CAD build for the part. Positions are in the model's coordinates, mm. Round coordinates to 2 decimals unless told otherwise and drop trailing zeros. Order: outer loops, then holes, each group sorted by start corner. A loop starts at its lowest first (then second) coordinate and runs counter-clockwise, first axis right, second up. Notation, with made-up numbers: (17.5, -32.75) - (31.5, -32.75) arc R21 cw to (31.5, -5.75) - close; hole circle Ø8 at (23, 6). An arc over 180 degrees is marked (long way). Use one line per item in the form item = value. Start each with the question number.
from build123d import *

# Parameters (mm, degrees)
SKETCH3_W           = 152.4
SKETCH3_H           = 152.4
BOSS_EXTRUDE1_DEPTH = 3.175
SKETCH4_R           = 11
CUT_EXTRUDE1_DEPTH  = 10
SKETCH5_R           = 3.175
CUT_EXTRUDE5_DEPTH  = 10


with BuildPart() as part:
    # Sketch3 → Boss-Extrude1 (new, symmetric)
    with BuildSketch(Plane(origin=(0, 0, 0), x_dir=(1, 0, 0), z_dir=(0, 1, 0))):
        Rectangle(SKETCH3_W, SKETCH3_H)
    extrude(amount=BOSS_EXTRUDE1_DEPTH, both=True)

    # Sketch4 → Cut-Extrude1 (cut)
    with BuildSketch(Plane(origin=(0, 3.175, 0), x_dir=(1, 0, 0), z_dir=(0, 1, 0))):
        with Locations(Location((-26.2, 26.2, 0), (0, 0, 270))):
            Circle(SKETCH4_R)
    extrude(amount=-CUT_EXTRUDE1_DEPTH, mode=Mode.SUBTRACT)

    # Sketch5 → Cut-Extrude5 (cut)
    with BuildSketch(Plane(origin=(0, 3.175, 0), x_dir=(1, 0, 0), z_dir=(0, 1, 0))):
        with Locations(Location((56.2, -35.2, 0), (0, 0, 270))):
            Circle(SKETCH5_R)
        with Locations(Location((56.2, -67.2, 0), (0, 0, 270))):
            Circle(SKETCH5_R)
    extrude(amount=-CUT_EXTRUDE5_DEPTH, mode=Mode.SUBTRACT)


solid = part.part
(1) Wall check: line 1 (X direction, y = 0, z = 35.2) (3 decimals); line 2 (X direction, y = -1, z = -26.2); line 3 (Z direction, x = -24, y = 1.5). Give the ranges that are in metal, low to high. Write a range as [from, to].
(2) Slice it at D-D (x = -26.2). Give the cut face in (y, z) (3 decimals), and give its area (3 significant figures).
(3) Slice it at A-A (x = 56.2). Give the cut face in (y, z) (3 decimals).
(4) Mould opens along X. For faces 1 (the flat face through (-1, 0, -76.2)), 2 (the flat face through (76.2, 0, 1)), 3 (the cylindrical face through (58.877, 0.044, 68.907)), 4 (the cylindrical face through (-36.94, 0.04, -28.58)) say: pulls with the +X half, pulls with the -X half, needs draft (parallel to the pull), parting line crosses it, or undercut.
(5) Slice it at C-C (y = 2). Give the cut face in (x, z) (3 decimals), and give its area (3 significant figures).
(6) Slice it at B-B (z = 35.2). Give the cut face in (x, y) (3 decimals).
Results list:
q1.line_1 = [-76.2, 53.025], [59.375, 76.2]
q1.line_2 = [-76.2, -37.2], [-15.2, 76.2]
q1.line_3 = [-76.2, -36.98], [-15.42, 76.2]
q2.outline = (-3.175, -76.2) - (3.175, -76.2) - (3.175, -37.2) - (-3.175, -37.2) - close; (-3.175, -15.2) - (3.175, -15.2) - (3.175, 76.2) - (-3.175, 76.2) - close
q2.area = 828 mm²
q3.outline = (-3.175, -76.2) - (3.175, -76.2) - (3.175, 32.025) - (-3.175, 32.025) - close; (-3.175, 38.375) - (3.175, 38.375) - (3.175, 64.025) - (-3.175, 64.025) - close; (-3.175, 70.375) - (3.175, 70.375) - (3.175, 76.2) - (-3.175, 76.2) - close
q4.face_1 = needs draft
q4.face_2 = pulls with the +X half
q4.face_3 = undercut
q4.face_4 = undercut
q5.outline = (-76.2, -76.2) - (76.2, -76.2) - (76.2, 76.2) - (-76.2, 76.2) - close; hole circle Ø22 at (-26.2, -26.2); hole circle Ø6.35 at (56.2, 35.2); hole circle Ø6.35 at (56.2, 67.2)
q5.area = 22,800 mm²
q6.outline = (-76.2, -3.175) - (53.025, -3.175) - (53.025, 3.175) - (-76.2, 3.175) - close; (59.375, -3.175) - (76.2, -3.175) - (76.2, 3.175) - (59.375, 3.175) - close
